Job drawing, mm, ordinate dimensions from the low corner. One solid piece. A direction names the side the tool comes from. Round coordinates to 2 decimals unless told otherwise and drop trailing zeros. Loops run counter-clockwise (first coordinate to the right, second up) from the corner with the lowest first, then second, coordinate; pieces in that order, holes last.
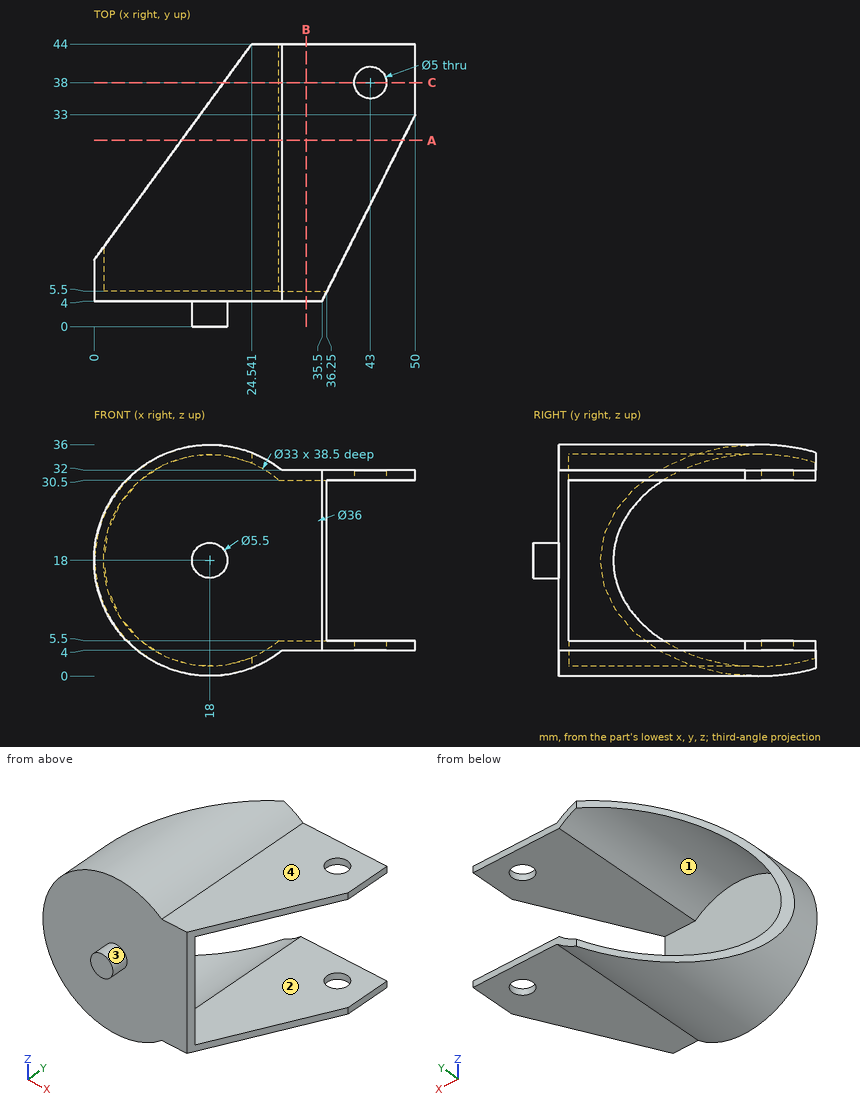
(1) Slice it at C-C on y = 38. List the corners of the cut face in (x, z).
Responses:
outline: (20.16, 0.13) arc R18 ccw to (29.31, 4) - (40.5, 4) - (40.5, 5.5) - (28.77, 5.5) arc R16.5 cw to (20.16, 1.64) - close; (20.16, 34.36) arc R16.5 cw to (28.77, 30.5) - (40.5, 30.5) - (40.5, 32) - (29.31, 32) arc R18 ccw to (20.16, 35.87) - close; (45.5, 4) - (50, 4) - (50, 5.5) - (45.5, 5.5) - close; (45.5, 30.5) - (50, 30.5) - (50, 32) - (45.5, 32) - close
(2) Pin check, flat tips, straight feed: P1, Ø10, axis at x = 21.5, y = 30, coming from the +Z side; P2, Ø2, axis at x = 42.5, y = 27, coming from the +Z side; P3, Ø4, axis at x = 24, y = 13, coming from the +Z side; P4, Ø4, axis at x = 43, y = 38, coming from the -Z side. Stop position of each tip, or through.
Responses:
P1: stops at z = 36
P2: stops at z = 32
P3: stops at z = 35.55
P4: passes through
(3) Which spindle directions (+Z, -Z, +X, -X, +Y, -Y) get a long thin tool onto all of the face, cutting with end or side? Do the marked faces 1, 2, 3 and 4. Say none if no direction does.
Responses:
face 1: +Y
face 2: +X, +Y
face 3: -Y
face 4: +Z, +X, +Y, -Y
(4) Slice it at B-B on x = 33. List the corners of the cut face in (y, z).
Responses:
outline: (4, 4) - (44, 4) - (44, 5.5) - (5.5, 5.5) - (5.5, 30.5) - (44, 30.5) - (44, 32) - (4, 32) - close
(5) Probe line 1 (Z direction, x = 32.5, y = 32.5); line 2 (Z direction, x = 28, y = 27) (1 decimal); line 3 (X direction, y = 38, z = 31). List the from-to ranges inside material, lowest first.
Responses:
line 1: z = 4 to 5.5, 30.5 to 32
line 2: z = 3 to 4.9, 31.1 to 33
line 3: x = 28.16 to 40.5, 45.5 to 50
(6) Slice it at A-A on y = 29. List the corners of the cut face in (x, z) (1 decimal), plus the area to 3 significant figures.
Responses:
outline: (13.6, 0.5) arc R18 ccw to (29.3, 4) - (48, 4) - (48, 5.5) - (28.8, 5.5) arc R16.5 cw to (13.6, 2.1) - close; (13.6, 33.9) arc R16.5 cw to (28.8, 30.5) - (48, 30.5) - (48, 32) - (29.3, 32) arc R18 ccw to (13.6, 35.5) - close
area: 106 mm2
